Could you check a few things on this model? Use its own coordinates, in mm. A direction names the side the tool comes from. Round coordinates to 2 decimals unless told otherwise and drop trailing zeros. Order: outer loops, then holes, each group sorted by start corner. A loop starts at its lowest first (then second) coordinate and runs counter-clockwise, first axis right, second up.
```python
from build123d import *

# Parameters (mm, degrees)
BOX311_W                    = 60
BOX311_H                    = 60
BOX311_DEPTH                = 7
BOX311_PLACEMENT_ANGLE      = 1
BOX312_W                    = 60
BOX312_H                    = 60
BOX312_DEPTH                = 7
BOX312_PLACEMENT_ANGLE      = 2
BOX310_W                    = 120
BOX310_H                    = 60
BOX310_DEPTH                = 7
TUBE084_R                   = 54.4
TUBE084_R_2                 = 53
TUBE084_DEPTH               = 7
BOX308_W                    = 60
BOX308_H                    = 60
BOX308_DEPTH                = 7
BOX308_PLACEMENT_ANGLE      = 20
BOX307_W                    = 60
BOX307_H                    = 60
BOX307_DEPTH                = 7
BOX307_PLACEMENT_ANGLE      = 20
BOX309_W                    = 120
BOX309_H                    = 60
BOX309_DEPTH                = 7
TUBE085_R                   = 54.4
TUBE085_R_2                 = 53
TUBE085_DEPTH               = 7
CUT335_PLACEMENT_ANGLE      = 225
CYLINDER804_R               = 52
CYLINDER804_DEPTH           = 7
BOX313_W                    = 1.4
BOX313_H                    = 60
BOX313_DEPTH                = 7
BOX313_PLACEMENT_ANGLE      = 2.7
BOX314_W                    = 1.4
BOX314_H                    = 60
BOX314_DEPTH                = 7
BOX314_PLACEMENT_ANGLE      = 2
CUT339_PLACEMENT_ANGLE      = 224.9
CYLINDER808_R               = 1.5
CYLINDER808_DEPTH           = 100
CYLINDER808_PLACEMENT_ANGLE = 100
CYLINDER806_R               = 1.5
CYLINDER806_DEPTH           = 100
CYLINDER806_PLACEMENT_ANGLE = 135
CYLINDER810_R               = 1.5
CYLINDER810_DEPTH           = 100
CYLINDER812_R               = 1.5
CYLINDER812_DEPTH           = 100
CYLINDER812_PLACEMENT_ANGLE = 225
CYLINDER805_R               = 1.5
CYLINDER805_DEPTH           = 100
CYLINDER809_R               = 1.5
CYLINDER809_DEPTH           = 100
CYLINDER809_PLACEMENT_ANGLE = 55
CYLINDER807_R               = 1.5
CYLINDER807_DEPTH           = 100
CYLINDER811_R               = 1.5
CYLINDER811_DEPTH           = 100
CYLINDER811_PLACEMENT_ANGLE = 45
TUBE087_R                   = 57
TUBE087_R_2                 = 30
TUBE087_DEPTH               = 10


with BuildPart() as krychle311:
    # Box311 → Box311 (new body)
    with BuildSketch(Plane.XY):
        with Locations((30, 30)):
            Rectangle(BOX311_W, BOX311_H)
    extrude(amount=BOX311_DEPTH)


with BuildPart() as krychle311_1:
    # Box311 placement: moved
    add(krychle311.part.moved(Location((-59.990862, -1.047144, -22))).rotate(Axis((-59.990862, -1.047144, -22), (0, 0, 1)), BOX311_PLACEMENT_ANGLE))


with BuildPart() as compound719:
    # Box312 → Box312 (new body)
    with BuildSketch(Plane.XY):
        with Locations((30, 30)):
            Rectangle(BOX312_W, BOX312_H)
    extrude(amount=BOX312_DEPTH)


with BuildPart() as compound719_1:
    # Box312 placement: moved
    add(compound719.part.moved(Location((0, 0, -22))).rotate(Axis((0, 0, -22), (0, 0, -1)), BOX312_PLACEMENT_ANGLE))

    # Compound719: union Krychle311
    add(krychle311_1.part)


with BuildPart() as krychle310:
    # Box310 → Box310 (new body)
    with BuildSketch(Plane(origin=(-60, -60, -22), x_dir=(1, 0, 0), z_dir=(0, 0, 1))):
        with Locations((60, 30)):
            Rectangle(BOX310_W, BOX310_H)
    extrude(amount=BOX310_DEPTH)


with BuildPart() as cut338:
    # Tube084 → Tube084 (new body)
    with BuildSketch(Plane.XY.offset(-22)):
        Circle(TUBE084_R)
        Circle(TUBE084_R_2, mode=Mode.SUBTRACT)
    extrude(amount=TUBE084_DEPTH)

    # Cut337: cut Krychle310
    add(krychle310.part, mode=Mode.SUBTRACT)

    # Cut338: cut Compound719
    add(compound719_1.part, mode=Mode.SUBTRACT)


with BuildPart() as cut338_1:
    # Cut338 placement: moved
    add(cut338.part.moved(Location((0, 0, -7))))


with BuildPart() as krychle308:
    # Box308 → Box308 (new body)
    with BuildSketch(Plane.XY):
        with Locations((30, 30)):
            Rectangle(BOX308_W, BOX308_H)
    extrude(amount=BOX308_DEPTH)


with BuildPart() as krychle308_1:
    # Box308 placement: moved
    add(krychle308.part.moved(Location((-56.381557, -20.521209, -22))).rotate(Axis((-56.381557, -20.521209, -22), (0, 0, 1)), BOX308_PLACEMENT_ANGLE))


with BuildPart() as compound718:
    # Box307 → Box307 (new body)
    with BuildSketch(Plane.XY):
        with Locations((30, 30)):
            Rectangle(BOX307_W, BOX307_H)
    extrude(amount=BOX307_DEPTH)


with BuildPart() as compound718_1:
    # Box307 placement: moved
    add(compound718.part.moved(Location((0, 0, -22))).rotate(Axis((0, 0, -22), (0, 0, -1)), BOX307_PLACEMENT_ANGLE))

    # Compound718: union Krychle308
    add(krychle308_1.part)


with BuildPart() as krychle309:
    # Box309 → Box309 (new body)
    with BuildSketch(Plane(origin=(-60, -60, -22), x_dir=(1, 0, 0), z_dir=(0, 0, 1))):
        with Locations((60, 30)):
            Rectangle(BOX309_W, BOX309_H)
    extrude(amount=BOX309_DEPTH)


with BuildPart() as cut335:
    # Tube085 → Tube085 (new body)
    with BuildSketch(Plane.XY.offset(-22)):
        Circle(TUBE085_R)
        Circle(TUBE085_R_2, mode=Mode.SUBTRACT)
    extrude(amount=TUBE085_DEPTH)

    # Cut334: cut Krychle309
    add(krychle309.part, mode=Mode.SUBTRACT)

    # Cut336: cut Compound718
    add(compound718_1.part, mode=Mode.SUBTRACT)


with BuildPart() as cut335_1:
    # Cut336 placement: moved
    add(cut335.part.moved(Location((0, 0, -7))))

    # Cut335: cut Cut338
    add(cut338_1.part, mode=Mode.SUBTRACT)


with BuildPart() as cut335_2:
    # Cut335 placement: moved
    add(cut335_1.part.moved(Location((0, 0, 74))).rotate(Axis((0, 0, 74), (0, 0, 1)), CUT335_PLACEMENT_ANGLE))


with BuildPart() as obj1:
    # Cylinder804 → Cylinder804 (new body)
    with BuildSketch(Plane.XY.offset(-22)):
        Circle(CYLINDER804_R)
    extrude(amount=CYLINDER804_DEPTH)


with BuildPart() as krychle313:
    # Box313 → Box313 (new body)
    with BuildSketch(Plane.XY):
        with Locations((0.7, 30)):
            Rectangle(BOX313_W, BOX313_H)
    extrude(amount=BOX313_DEPTH)


with BuildPart() as krychle313_1:
    # Box313 placement: moved
    add(krychle313.part.moved(Location((0, 0, -22))).rotate(Axis((0, 0, -22), (0, 0, 1)), BOX313_PLACEMENT_ANGLE))


with BuildPart() as cut339:
    # Box314 → Box314 (new body)
    with BuildSketch(Plane.XY):
        with Locations((0.7, 30)):
            Rectangle(BOX314_W, BOX314_H)
    extrude(amount=BOX314_DEPTH)


with BuildPart() as cut339_1:
    # Box314 placement: moved
    add(cut339.part.moved(Location((0, 0, -22))).rotate(Axis((0, 0, -22), (0, 0, -1)), BOX314_PLACEMENT_ANGLE))

    # Compound720: union Krychle313
    add(krychle313_1.part)

    # Cut339: cut obj1
    add(obj1.part, mode=Mode.SUBTRACT)


with BuildPart() as cut339_2:
    # Cut339 placement: moved
    add(cut339_1.part.moved(Location((0, 0, 67))).rotate(Axis((0, 0, 67), (0, 0, 1)), CUT339_PLACEMENT_ANGLE))


with BuildPart() as obj2:
    # Cylinder808 → Cylinder808 (new body)
    with BuildSketch(Plane.XY):
        Circle(CYLINDER808_R)
    extrude(amount=CYLINDER808_DEPTH)


with BuildPart() as obj2_1:
    # Cylinder808 placement: moved
    add(obj2.part.moved(Location((41.004432, -9.090464, 0))).rotate(Axis((41.004432, -9.090464, 0), (0, 0, 1)), CYLINDER808_PLACEMENT_ANGLE))


with BuildPart() as obj3:
    # Cylinder806 → Cylinder806 (new body)
    with BuildSketch(Plane.XY):
        Circle(CYLINDER806_R)
    extrude(amount=CYLINDER806_DEPTH)


with BuildPart() as obj3_1:
    # Cylinder806 placement: moved
    add(obj3.part.moved(Location((38.80294, 16.072704, 0))).rotate(Axis((38.80294, 16.072704, 0), (0, 0, 1)), CYLINDER806_PLACEMENT_ANGLE))


with BuildPart() as obj4:
    # Cylinder810 → Cylinder810 (new body)
    with BuildSketch(Plane(origin=(16.072704, 38.80294, 0), x_dir=(-1, 0, 0), z_dir=(0, 0, 1))):
        Circle(CYLINDER810_R)
    extrude(amount=CYLINDER810_DEPTH)


with BuildPart() as obj5:
    # Cylinder812 → Cylinder812 (new body)
    with BuildSketch(Plane.XY):
        Circle(CYLINDER812_R)
    extrude(amount=CYLINDER812_DEPTH)


with BuildPart() as obj5_1:
    # Cylinder812 placement: moved
    add(obj5.part.moved(Location((-16.072704, 38.80294, 0))).rotate(Axis((-16.072704, 38.80294, 0), (0, 0, 1)), CYLINDER812_PLACEMENT_ANGLE))


with BuildPart() as obj6:
    # Cylinder805 → Cylinder805 (new body)
    with BuildSketch(Plane(origin=(-38.80294, 16.072704, 0), x_dir=(0, -1, 0), z_dir=(0, 0, 1))):
        Circle(CYLINDER805_R)
    extrude(amount=CYLINDER805_DEPTH)


with BuildPart() as obj7:
    # Cylinder809 → Cylinder809 (new body)
    with BuildSketch(Plane.XY):
        Circle(CYLINDER809_R)
    extrude(amount=CYLINDER809_DEPTH)


with BuildPart() as obj7_1:
    # Cylinder809 placement: moved
    add(obj7.part.moved(Location((-41.004432, -9.090464, 0))).rotate(Axis((-41.004432, -9.090464, 0), (0, 0, -1)), CYLINDER809_PLACEMENT_ANGLE))


with BuildPart() as obj8:
    # Cylinder807 → Cylinder807 (new body)
    with BuildSketch(Plane(origin=(-16.072704, -38.80294, 0), x_dir=(1, 0, 0), z_dir=(0, 0, 1))):
        Circle(CYLINDER807_R)
    extrude(amount=CYLINDER807_DEPTH)


with BuildPart() as compound721:
    # Cylinder811 → Cylinder811 (new body)
    with BuildSketch(Plane.XY):
        Circle(CYLINDER811_R)
    extrude(amount=CYLINDER811_DEPTH)


with BuildPart() as compound721_1:
    # Cylinder811 placement: moved
    add(compound721.part.moved(Location((16.072704, -38.80294, 0))).rotate(Axis((16.072704, -38.80294, 0), (0, 0, 1)), CYLINDER811_PLACEMENT_ANGLE))

    # Compound721: union obj2, obj3, obj4, obj5, obj6, obj7, obj8
    add(obj2_1.part)
    add(obj3_1.part)
    add(obj4.part)
    add(obj5_1.part)
    add(obj6.part)
    add(obj7_1.part)
    add(obj8.part)


with BuildPart() as cut342:
    # Tube087 → Tube087 (new body)
    with BuildSketch(Plane.XY.offset(42)):
        Circle(TUBE087_R)
        Circle(TUBE087_R_2, mode=Mode.SUBTRACT)
    extrude(amount=TUBE087_DEPTH)

    # Cut340: cut Compound721
    add(compound721_1.part, mode=Mode.SUBTRACT)

    # Cut341: cut Cut339
    add(cut339_2.part, mode=Mode.SUBTRACT)

    # Cut342: cut Cut335
    add(cut335_2.part, mode=Mode.SUBTRACT)


solid = cut342.part
```
Q1. For faces 4 (the cylindrical face through (45.194, -30.28, 48.451)), 5 (the cylindrical face through (42.5, -9.2, 46.9)), which set-ups out of +Z, -Z, +X, -X, +Y, -Y let a thin tool reach every point of the face, with its end or its side?
Q2. Imagine slicing it at A-A, the plane x = 0. Please give me the cut outline in (y, z).
Q3. For P1, Ø1.8, axis at x = 16.07, y = 38.8, coming from the +Z side; P2, Ø2, axis at y = -18.5, z = 46, coming from the -X side; P3, Ø1, axis at x = -43.5, z = 44.5, coming from the -Y side; P4, Ø1.5, axis at x = -23.5, z = 44, coming from the -Y side, each with a flat end and sliding along its axis, tell me the tip position at first contact or that it passes through.
Q4. Imagine slicing it at C-C, the plane z = 47. State how many separate pieces and enclosed holes the cut face has, then the cut area to 3 significant figures.
Q5. We'd pull the mould along Y, two halves only. Please class faces 1 (the flat face through (25, -25, 42)), 2 (the flat face through (31, -44, 45)), 3 (the cylindrical face through (52.654, -21.831, 46.93)): released by +Y, released by -Y, zero draft, split by the parting line, or undercut.
Q6. I need wall thicknesses on L1, parallel to X at y = -37.5, z = 44.25; L2, parallel to Y at x = 0, z = 49; L3, parallel to X at y = -1, z = 45.75. Which ranges of each line are inside material? Lowest first, please.
Filled in:
1. face 4: +Z
1. face 5: +Z, -Z
2. outline: (-57, 42) - (-30, 42) - (-30, 52) - (-57, 52) - close; (30, 42) - (57, 42) - (57, 52) - (30, 52) - close
3. P1: passes through
3. P2: stops at x = -54.25
3. P3: stops at y = -37.42
3. P4: stops at y = -52.26
4. separate pieces: 1
4. enclosed holes: 9
4. area: 7,260 mm2
5. face 1: zero draft
5. face 2: undercut
5. face 3: split by the parting line
6. L1: x = -42.93 to -16.82, -15.33 to 15.33, 16.82 to 42.93
6. L2: y = -57 to -30, 30 to 57
6. L3: x = -56.99 to -29.98, 29.98 to 56.99
